For this review, take the finished solid that the model builds, in its own axes (mm). Round coordinates to 2 decimals unless told otherwise and drop trailing zeros. Loops run counter-clockwise (first coordinate to the right, second up) from the corner with the lowest first, then second, coordinate; pieces in that order, holes last.
Autodesk Inventor part; units mm, degrees
ref_plane "YZ Plane" through (0, 0, 0) normal (1, 0, 0) x (0, 1, 0)
ref_plane "XZ Plane" through (0, 0, 0) normal (0, 1, 0) x (-1, 0, 0)
ref_plane "XY Plane" through (0, 0, 0) normal (0, 0, 1) x (1, 0, 0)
sketch "スケッチ1" plane through (0, 0, 0) normal (0, 0, 1) x (1, 0, 0)
  line L0 (-23.5, -3.5) -> (23.5, -3.5)
  line L1 (23.5, -3.5) -> (23.5, 3.5) construction
  line L2 (23.5, 3.5) -> (-23.5, 3.5)
  line L3 (-23.5, 3.5) -> (-23.5, -3.5) construction
  line L4 (-23.5, -3.5) -> (23.5, 3.5) construction
  line L5 (23.5, -3.5) -> (-23.5, 3.5) construction
  circle A0 centre (-23.5, 0) radius 3.5
  line L6 (0, 3.5) -> (0, -3.5) construction
  circle A1 centre (23.5, 0) radius 3.5
  circle A2 centre (-23.5, 0) radius 2.25
  circle A3 centre (23.5, 0) radius 2.25
  point P0 (0, 0)
  point P1 (23.5, -3.5)
  point P2 (23.5, 3.5)
  dimension "d0" = 7
  dimension "d1" = 47
  dimension "d2" = 4.5
extrude "押し出し1" add sketch "スケッチ1" along normal blind 1.5
sketch "スケッチ2" plane through (0, 0, 1.5) normal (0, 0, 1) x (1, 0, 0)
  circle A0 centre (23.5, 0) radius 2.25 construction
  circle A1 centre (-23.5, 0) radius 2.25 construction
  line L0 (23.5, 0) -> (-23.5, 0) construction
  circle A2 centre (0, 0) radius 1.1
  circle A3 centre (-5, 0) radius 1.1
  circle A4 centre (-10, 0) radius 1.1
  circle A5 centre (-15, 0) radius 1.1
  circle A6 centre (-20, 0) radius 1.1
  circle A7 centre (5, 0) radius 1.1
  circle A8 centre (0, 0) radius 1.1
  circle A9 centre (-5, 0) radius 1.1
  circle A10 centre (-10, 0) radius 1.1
  circle A11 centre (-15, 0) radius 1.1
  circle A12 centre (10, 0) radius 1.1
  circle A13 centre (5, 0) radius 1.1
  circle A14 centre (0, 0) radius 1.1
  circle A15 centre (-5, 0) radius 1.1
  circle A16 centre (-10, 0) radius 1.1
  circle A17 centre (15, 0) radius 1.1
  circle A18 centre (10, 0) radius 1.1
  circle A19 centre (5, 0) radius 1.1
  circle A20 centre (0, 0) radius 1.1
  circle A21 centre (-5, 0) radius 1.1
  circle A22 centre (20, 0) radius 1.1
  circle A23 centre (15, 0) radius 1.1
  circle A24 centre (10, 0) radius 1.1
  circle A25 centre (5, 0) radius 1.1
  circle A26 centre (0, 0) radius 1.1
  dimension "d5" = 2.2
  dimension "d8" = 5
  dimension "d11" = 5
extrude "押し出し2" cut sketch "スケッチ2" against normal through all contours A2 | A3 | A7
properties part number "free_link" material "アルミニウム 2014-T4"
(1) Add section C-C (z = 0.35). Give the boundary of the cut face in (x, y), plus the area to 3 significant figures.
(2) Insertion check: pin 1 Ø4 at (x, y) = (12.5, -0.5) entering from -Z; pin 2 Ø1.8 at (x, y) = (0, 0) entering from -Z. Each pin has a flat end and moves straight along its axis. Give the tip position at first contact, or say it passes through.
(3) Add section B-B (x = -5). Give the boundary of the cut face in (y, z).
(4) For L1, parallel to Y at x = 5, z = 1.15; L2, parallel to Y at x = -23.5, z = 0.4; L3, parallel to X at y = -1, z = 0.45, list the stretches that pass through material, from the lowest coordinate up.
(5) The part is to be moulded in two halves that separate along X. For faces 1 (the cylindrical face through (-3.95, 0.33, 0.76)), 2 (the cylindrical face through (-27, 0, 1)), 3 (the cylindrical face through (27, 0, 1)), say which applies: pulls with the +X half, pulls with the -X half, needs draft (parallel to the pull), parting line crosses it, or undercut.
(6) Add section A-A (y = 0). Give the boundary of the cut face in (x, z).
Outcome:
1. outline: (-23.5, -3.5) - (23.5, -3.5) arc R3.5 ccw to (23.5, 3.5) - (-23.5, 3.5) arc R3.5 ccw to start; hole circle Ø4.5 at (-23.5, 0); hole circle Ø2.2 at (-5, 0); hole circle Ø2.2 at (0, 0); hole circle Ø2.2 at (5, 0); hole circle Ø4.5 at (23.5, 0)
1. area: 324 mm2
2. pin 1: stops at z = 0
2. pin 2: passes through
3. outline: (-3.5, 0) - (-1.1, 0) - (-1.1, 1.5) - (-3.5, 1.5) - close; (1.1, 0) - (3.5, 0) - (3.5, 1.5) - (1.1, 1.5) - close
4. L1: y = -3.5 to -1.1, 1.1 to 3.5
4. L2: y = -3.5 to -2.25, 2.25 to 3.5
4. L3: x = -26.85 to -25.52, -21.48 to -5.46, -4.54 to -0.46, 0.46 to 4.54, 5.46 to 21.48, 25.52 to 26.85
5. face 1: undercut
5. face 2: pulls with the -X half
5. face 3: pulls with the +X half
6. outline: (-27, 0) - (-25.75, 0) - (-25.75, 1.5) - (-27, 1.5) - close; (-21.25, 0) - (-6.1, 0) - (-6.1, 1.5) - (-21.25, 1.5) - close; (-3.9, 0) - (-1.1, 0) - (-1.1, 1.5) - (-3.9, 1.5) - close; (1.1, 0) - (3.9, 0) - (3.9, 1.5) - (1.1, 1.5) - close; (6.1, 0) - (21.25, 0) - (21.25, 1.5) - (6.1, 1.5) - close; (25.75, 0) - (27, 0) - (27, 1.5) - (25.75, 1.5) - close
